Geometry: final body of the model. Coordinates: model frame, mm. Face numbers are marked on the shaded views. A direction names the side the tool comes from. Give positions to 0.01 mm unless a question says otherwise; leave off trailing zeros. Loops run counter-clockwise (first coordinate to the right, second up) from the corner with the lowest first, then second, coordinate; pieces in that order, holes last.
1. Access query for the marked faces 1 and 2. Directions: +Z, -Z, +X, -X, +Y, -Y. A direction counts if a zero-diameter tool reaches every point of the face in a straight line with its end or side. Return the directions, or none.
2. Material intervals for line 1 along X through (y, z) = (-0.6, -19.05) (3 decimals); line 2 along Z through (x, y) = (19.05, -1.6) (3 decimals); line 3 along Y through (x, z) = (180.5, -28.5), sorted ascending.
3. Section A-A, the plane x = 353.5. Output: boundary loops of the cut face in (y, z), then the cut area to 3 significant figures.
4. Section B-B, the plane z = -29.5. Output: boundary loops of the cut face in (x, y).
5. Section C-C, the plane y = 27. Output: boundary loops of the cut face in (x, z), then the cut area to 3 significant figures.
6. First-contact query: P1, Ø1.5, axis at y = 2.5, z = -18.5, coming from the -X side; P2, Ø1.5, axis at x = 209.5, z = -4.5, coming from the +Y side; P3, Ø10, axis at x = 347, y = 15, coming from the +Z side. Flat tips, straight axial feed; report the tip coordinate or a pass-through.
from build123d import *

# Parameters (mm, degrees)
SKETCH1_W                    = 444.5
SKETCH1_H                    = 38.1
BASE_FLANGE1_DEPTH           = 2.304796
EDGE_FLANGE1_STRIP_W         = 14.299184
EDGE_FLANGE1_STRIP_H         = 2.304796
EDGE_FLANGE1_STRIP_CUT_DEPTH = 444.5
EDGE_FLANGE1_DEPTH           = 444.5
F_1_4_0_25_DIAMETER_HOLE1_D  = 6.35


# Sheet-metal steps are written as plain solids
with BuildPart() as part:
    # Sketch1 → Base-Flange1 (new body)
    with BuildSketch(Plane(origin=(0, 0, 0), x_dir=(1, 0, 0), z_dir=(0, 1, 0))):
        with Locations((222.25, 19.05)):
            Rectangle(SKETCH1_W, SKETCH1_H)
    extrude(amount=-BASE_FLANGE1_DEPTH)

    # Edge-Flange1 strip (across the edge) → Edge-Flange1 strip cut (cut)
    with BuildSketch(Plane(origin=(444.5, 0, -38.1), x_dir=(0, 0, 1), z_dir=(-1, 0, 0))):
        with Locations((-2.304796, -1.152398)):
            Rectangle(EDGE_FLANGE1_STRIP_W, EDGE_FLANGE1_STRIP_H)
    extrude(amount=EDGE_FLANGE1_STRIP_CUT_DEPTH, mode=Mode.SUBTRACT)

    # Edge-Flange1 section (across the edge) → Edge-Flange1 (add)
    with BuildSketch(Plane(origin=(444.5, 0, -38.1), x_dir=(0, 0, 1), z_dir=(-1, 0, 0))):
        with BuildLine():
            Line((0, 2.54), (0, 35.795204))
            Line((0, 35.795204), (2.304796, 35.795204))
            Line((2.304796, 35.795204), (2.304796, 2.54))
            ThreePointArc((2.304796, 2.54), (3.048744776, 0.743948776), (4.844796, 0))
            Line((4.844796, 0), (4.844796, -2.304796))
            ThreePointArc((4.844796, -2.304796), (1.419007895, -0.885788105), (0, 2.54))
        make_face()
    extrude(amount=EDGE_FLANGE1_DEPTH)

    # 1/4 (0.25) Diameter Hole1 (through all)
    with Locations(Plane(origin=(0, 0, 0), x_dir=(1, 0, 0), z_dir=(0, 1, 0))):
        with Locations((19.05, 19.05), (425.45, 19.05)):
            Hole(F_1_4_0_25_DIAMETER_HOLE1_D / 2)


solid = part.part
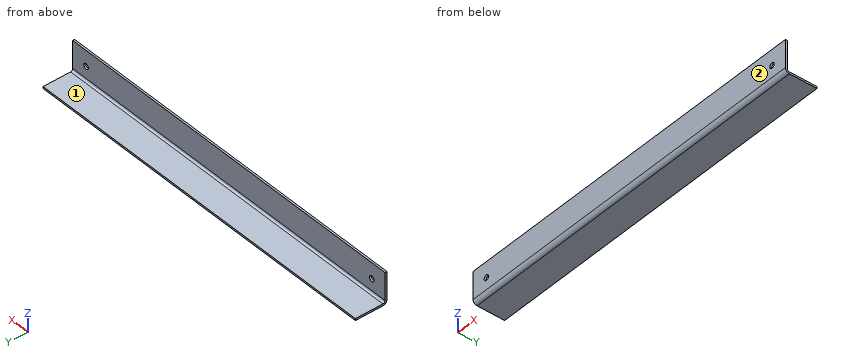
Answers below:
1. face 1: +Z, +X, -X, +Y
1. face 2: +Z, -Z, +X, -X, -Y
2. line 1: x = 0 to 15.875, 22.225 to 422.275, 428.625 to 444.5
2. line 2: z = -35.772 to -22.225, -15.875 to 0
2. line 3: y = -2.3 to 0
3. outline: (-2.3, -33.26) arc R4.84 ccw to (2.54, -38.1) - (35.8, -38.1) - (35.8, -35.8) - (2.54, -35.8) arc R2.54 cw to (0, -33.26) - (0, 0) - (-2.3, 0) - close
3. area: 167 mm2
4. outline: (0, -2.3) - (444.5, -2.3) - (444.5, 0) - (0, 0) - close
5. outline: (0, -38.1) - (444.5, -38.1) - (444.5, -35.8) - (0, -35.8) - close
5. area: 1,020 mm2
6. P1: passes through
6. P2: stops at y = 0
6. P3: stops at z = -35.8
